The figure shows three views and two pictorial views of one solid part (mm, origin at its lowest corner). Answer the questions. A direction names the side the tool comes from. Round coordinates to 2 decimals unless told otherwise and drop trailing zeros. Loops run counter-clockwise (first coordinate to the right, second up) from the corner with the lowest first, then second, coordinate; pieces in that order, holes last. Notation, with made-up numbers: (-30, 50) -> (-15, 50) arc R10 ccw to (-15, 61) -> close; hole circle Ø8 at (86.25, 70.25). An arc over 180 degrees is marked (long way). Write each question's results on one line, items separated by ' | '. Start each with the question number.
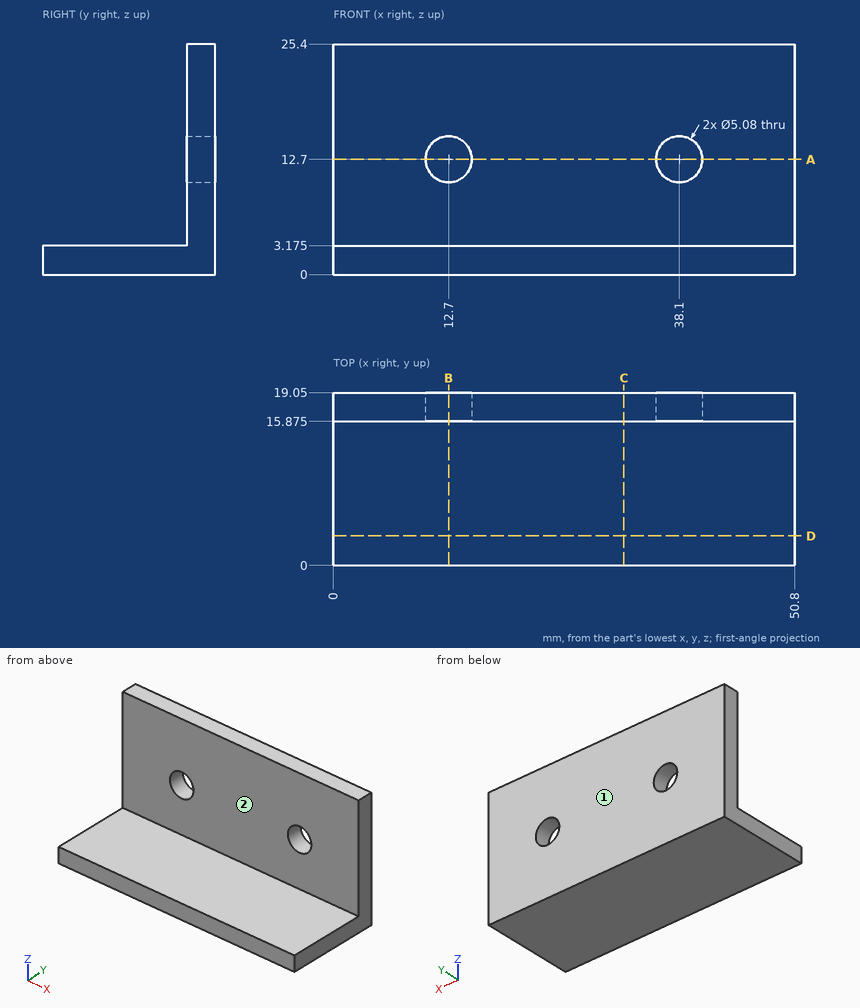
Item 1: The part is cut by section D-D, the plane y = 3.25. Give the vertices of the cut face in (x, z) (3 decimals).
Item 2: For the marked faces 1 and 2, determine the directions among +Z, -Z, +X, -X, +Y, -Y from which every point of the face is accessible in a straight line to the end or side of a thin tool.
Item 3: Each of these flat-tipped pins is pushed along its axis until it touches: pin 1 Ø2 at (x, z) = (27.5, 2.5) entering from -Y; pin 2 Ø6.5 at (x, z) = (38.1, 12.7) entering from -Y (3 decimals); pin 3 Ø1 at (x, z) = (13.5, 11) entering from -Y. Where does it stop, or does it pass through?
Item 4: Straight lines are drawn through the part: L1, parallel to X at y = 17.3, z = 12.7; L2, parallel to Z at x = 12.7, y = 18.05; L3, parallel to Y at x = 19.5, z = 13.5 (3 decimals). For each, find the intervals that lie inside material, in ascending order. Write a range as [from, to].
Item 5: The part is cut by section B-B, the plane x = 12.7. Give the vertices of the cut face in (y, z) (3 decimals).
Item 6: The part is cut by section A-A, the plane z = 12.7. Give the vertices of the cut face in (x, y) (3 decimals).
Item 7: The part is cut by section C-C, the plane x = 32. Give the vertices of the cut face in (y, z) (3 decimals), plus the area to 3 significant figures.
Report:
1) outline: (0, 0) -> (50.8, 0) -> (50.8, 3.175) -> (0, 3.175) -> close
2) face 1: +Z, -Z, +X, -X, +Y | face 2: +Z, +X, -X, -Y
3) pin 1: stops at y = 0 | pin 2: stops at y = 15.875 | pin 3: passes through
4) L1: x = [0, 10.16], [15.24, 35.56], [40.64, 50.8] | L2: z = [0, 10.16], [15.24, 25.4] | L3: y = [15.875, 19.05]
5) outline: (0, 0) -> (19.05, 0) -> (19.05, 10.16) -> (15.875, 10.16) -> (15.875, 3.175) -> (0, 3.175) -> close; (15.875, 15.24) -> (19.05, 15.24) -> (19.05, 25.4) -> (15.875, 25.4) -> close
6) outline: (0, 15.875) -> (10.16, 15.875) -> (10.16, 19.05) -> (0, 19.05) -> close; (15.24, 15.875) -> (35.56, 15.875) -> (35.56, 19.05) -> (15.24, 19.05) -> close; (40.64, 15.875) -> (50.8, 15.875) -> (50.8, 19.05) -> (40.64, 19.05) -> close
7) outline: (0, 0) -> (19.05, 0) -> (19.05, 25.4) -> (15.875, 25.4) -> (15.875, 3.175) -> (0, 3.175) -> close | area: 131 mm2
